Work out the finished part from the listing and answer in its coordinate system (mm). Face numbers are marked on the shaded views. A direction names the side the tool comes from. Give positions to 0.01 mm unless a question says otherwise; leave off trailing zeros. Order: outer loops, then holes, each group sorted by start corner. A loop starts at its lowest first (then second) coordinate and runs counter-clockwise, first axis right, second up.
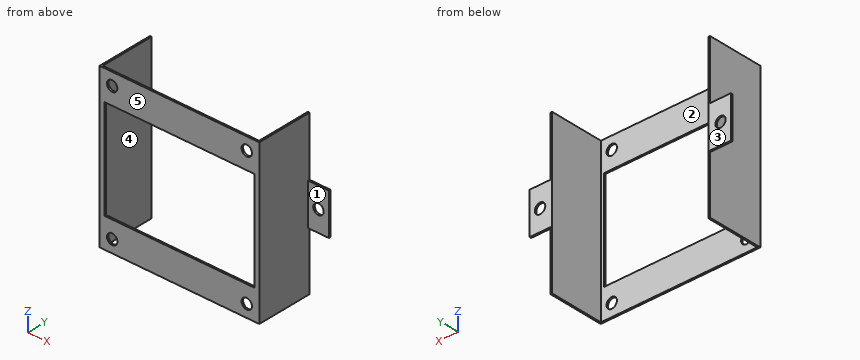
```python
from build123d import *

# Parameters (mm, degrees)
SKETCH_1_W          = 75
SKETCH_1_H          = 75
EXTRUDE_1_DEPTH     = 0.8
SKETCH_2_W          = 76.6
SKETCH_2_H          = 76.6
SKETCH_2_W_2        = 75
SKETCH_2_H_2        = 75
EXTRUDE_2_DEPTH     = 26.8
SKETCH_3_W          = 10.8
SKETCH_3_H          = 20
EXTRUDE_3_DEPTH     = 0.8
F_5_0MM_1_D         = 5
SKETCH_6_W          = 75
SKETCH_6_H          = 26
CUT_EXTRUDE_1_DEPTH = 119.099280269
F_5_0MM_2_D         = 5


with BuildPart() as part:
    # 草图1 → 凸台-拉伸1 (new body)
    with BuildSketch(Plane(origin=(0, 0, 0), x_dir=(1, 0, 0), z_dir=(0, 1, 0))):
        with Locations((37.5, -37.5)):
            Rectangle(SKETCH_1_W, SKETCH_1_H)
        Polygon((73.5, -37.5), (73.5, -13.5), (1.5, -13.5), (1.5, -61.5), (73.5, -61.5), align=None, mode=Mode.SUBTRACT)
    extrude(amount=EXTRUDE_1_DEPTH)

    # 草图2 → 凸台-拉伸2 (add)
    with BuildSketch(Plane.XZ):
        with Locations((37.5, 37.5)):
            Rectangle(SKETCH_2_W, SKETCH_2_H)
        with Locations((37.5, 37.5)):
            Rectangle(SKETCH_2_W_2, SKETCH_2_H_2, mode=Mode.SUBTRACT)
    extrude(amount=-EXTRUDE_2_DEPTH)

    # 草图3 → 凸台-拉伸3 (add)
    with BuildSketch(Plane(origin=(0, 26.8, 0), x_dir=(1, 0, 0), z_dir=(0, 1, 0))):
        with Locations((-5.4, -37.5)):
            Rectangle(SKETCH_3_W, SKETCH_3_H)
        with Locations((80.4, -37.5)):
            Rectangle(SKETCH_3_W, SKETCH_3_H)
    extrude(amount=-EXTRUDE_3_DEPTH)

    # Ø5.0mm 暗销孔1 (through all)
    with Locations(Plane(origin=(0, 26.8, 0), x_dir=(1, 0, 0), z_dir=(0, 1, 0))):
        with Locations((80.8, -37.5), (-5.8, -37.5)):
            Hole(F_5_0MM_1_D / 2)

    # 草图6 → 切除-拉伸1 (cut, through all)
    with BuildSketch(Plane.XY.offset(75.8)):
        with Locations((37.5, 13.8)):
            Rectangle(SKETCH_6_W, SKETCH_6_H)
    extrude(amount=-CUT_EXTRUDE_1_DEPTH, mode=Mode.SUBTRACT)

    # Ø5.0mm 暗销孔2 (through all)
    with Locations(Plane(origin=(0, 0, 0), x_dir=(-1, 0, 0), z_dir=(0, -1, 0))):
        with Locations((-69.8, -69.8), (-69.8, -5.2), (-5.2, -5.2), (-5.2, -69.8)):
            Hole(F_5_0MM_2_D / 2)


solid = part.part
```
1. Which of the six approach directions +Z, -Z, +X, -X, +Y, -Y give full straight-line access (tool end or side, diameter ignored) to the marked faces 1, 2 and 3?
Findings below:
face 1: +Z, -Z, +X, -Y
face 2: +Z, -Z, +Y
face 3: +Z, -Z, +X, -X, +Y
2. Straight lines are drawn through the part: probe 1 along Z at (x, y) = (69.8, 0.2); probe 2 along X at (y, z) = (24.5, 4); probe 3 along X at (y, z) = (0.3, 69.8). For each, find the intervals that lie inside material, in ascending order.
Findings below:
probe 1: z = -0.8 to 2.7, 7.7 to 13.5, 61.5 to 67.3, 72.3 to 75.8
probe 2: x = -0.8 to 0, 75 to 75.8
probe 3: x = -0.8 to 2.7, 7.7 to 67.3, 72.3 to 75.8
3. The part is cut by section C-C (y = 4.5). Write down the section's boundary in (x, z), then the cut area to 3 significant figures.
Findings below:
outline: (-0.8, -0.8) - (0, -0.8) - (0, 75.8) - (-0.8, 75.8) - close; (75, -0.8) - (75.8, -0.8) - (75.8, 75.8) - (75, 75.8) - close
area: 123 mm2
4. The part is cut by section A-A (z = 69.8). Write down the section's boundary in (x, y).
Findings below:
outline: (-0.8, 0) - (2.7, 0) - (2.7, 0.8) - (0, 0.8) - (0, 26.8) - (-0.8, 26.8) - close; (7.7, 0) - (67.3, 0) - (67.3, 0.8) - (7.7, 0.8) - close; (72.3, 0) - (75.8, 0) - (75.8, 26.8) - (75, 26.8) - (75, 0.8) - (72.3, 0.8) - close
5. Given P1, Ø3, axis at x = 5.2, z = 5.2, coming from the +Y side; P2, Ø12, axis at y = 10.5, z = 61.5, coming from the -X side; P3, Ø6.5, axis at x = 69.8, z = 69.8, coming from the +Y side; P4, Ø6.5, axis at x = 80.8, z = 37.5, coming from the -Y side, each flat-ended and moving along its own axis, determine where each tip first touches the part or whether it passes through.
Findings below:
P1: passes through
P2: stops at x = -0.8
P3: stops at y = 0.8
P4: stops at y = 26
6. The part is cut by section D-D (z = 37.5). Write down the section's boundary in (x, y), then the cut area to 3 significant figures.
Findings below:
outline: (-10.8, 26) - (-8.3, 26) - (-8.3, 26.8) - (-10.8, 26.8) - close; (-3.3, 26) - (-0.8, 26) - (-0.8, 0) - (1.5, 0) - (1.5, 0.8) - (0, 0.8) - (0, 26.8) - (-3.3, 26.8) - close; (73.5, 0) - (75.8, 0) - (75.8, 26) - (78.3, 26) - (78.3, 26.8) - (75, 26.8) - (75, 0.8) - (73.5, 0.8) - close; (83.3, 26) - (85.8, 26) - (85.8, 26.8) - (83.3, 26.8) - close
area: 53.3 mm2
7. The part is cut by section B-B (x = -5.8). Write down the section's boundary in (y, z), then the cut area to 3 significant figures.
Findings below:
outline: (26, 27.5) - (26.8, 27.5) - (26.8, 35) - (26, 35) - close; (26, 40) - (26.8, 40) - (26.8, 47.5) - (26, 47.5) - close
area: 12.0 mm2
8. The mould has two halves that part along X. Classify the marked faces 4 and 5: pulls with the +X half, pulls with the -X half, needs draft (parallel to the pull), parting line crosses it, or undercut.
Findings below:
face 4: undercut
face 5: needs draft
